```python
from build123d import *

# Parameters (mm, degrees)
SKETCH1_W           = 384
SKETCH1_H           = 140
SKETCH1_R           = 4
SKETCH1_R_2         = 3
BOSS_EXTRUDE1_DEPTH = 3
FILLET1_R           = 3


with BuildPart() as part:
    # Sketch1 → Boss-Extrude1 (new body)
    with BuildSketch(Plane(origin=(0, 0, 0), x_dir=(1, 0, 0), z_dir=(0, 1, 0))):
        Rectangle(SKETCH1_W, SKETCH1_H)
        with Locations(Location((-34, 56, 0), (0, 0, 270))):
            Circle(SKETCH1_R, mode=Mode.SUBTRACT)
        with Locations(Location((-39.2, 10, 0), (0, 0, 270))):
            Circle(SKETCH1_R, mode=Mode.SUBTRACT)
        with Locations(Location((0, -56, 0), (0, 0, 270))):
            Circle(SKETCH1_R, mode=Mode.SUBTRACT)
        with Locations(Location((39.2, 10, 0), (0, 0, 90))):
            Circle(SKETCH1_R, mode=Mode.SUBTRACT)
        with Locations(Location((34, 56, 0), (0, 0, 90))):
            Circle(SKETCH1_R, mode=Mode.SUBTRACT)
        with Locations(Location((-178, -56, 0), (0, 0, 270))):
            Circle(SKETCH1_R_2, mode=Mode.SUBTRACT)
        with Locations(Location((178, -56, 0), (0, 0, 90))):
            Circle(SKETCH1_R_2, mode=Mode.SUBTRACT)
        with Locations(Location((-178, 56, 0), (0, 0, 90))):
            Circle(SKETCH1_R_2, mode=Mode.SUBTRACT)
        with Locations(Location((178, 56, 0), (0, 0, 270))):
            Circle(SKETCH1_R_2, mode=Mode.SUBTRACT)
        with Locations(Location((-178, 18.666666667, 0), (0, 0, 270))):
            Circle(SKETCH1_R_2, mode=Mode.SUBTRACT)
        with Locations(Location((-178, -18.666666667, 0), (0, 0, 90))):
            Circle(SKETCH1_R_2, mode=Mode.SUBTRACT)
        with Locations(Location((178, 18.666666667, 0), (0, 0, 90))):
            Circle(SKETCH1_R_2, mode=Mode.SUBTRACT)
        with Locations(Location((178, -18.666666667, 0), (0, 0, 270))):
            Circle(SKETCH1_R_2, mode=Mode.SUBTRACT)
        with BuildLine():
            Line((-28.508169209, 15.556618484), (-26.070198724, 37.123280462))
            ThreePointArc((-26.070198724, 37.123280462), (-22.795588541, 43.457640532), (-16.133486944, 46))
            Line((-16.133486944, 46), (16.133486944, 46))
            ThreePointArc((16.133486944, 46), (22.795588541, 43.457640532), (26.070198724, 37.123280462))
            Line((26.070198724, 37.123280462), (28.508169209, 15.556618484))
            ThreePointArc((28.508169209, 15.556618484), (28.348223714, 12.33218572), (27.169289942, 9.326746589))
            Line((27.169289942, 9.326746589), (8.597832514, -21.941523571))
            ThreePointArc((8.597832514, -21.941523571), (0, -26.834932138), (-8.597832514, -21.941523571))
            Line((-8.597832514, -21.941523571), (-27.169289942, 9.326746589))
            ThreePointArc((-27.169289942, 9.326746589), (-28.348223714, 12.33218572), (-28.508169209, 15.556618484))
        make_face(mode=Mode.SUBTRACT)
    extrude(amount=BOSS_EXTRUDE1_DEPTH)

    # Fillet1
    fillet1_edges = [part.edges().sort_by_distance(p)[0] for p in [
        (192, 1.5, 70),
        (-192, 1.5, 70),
        (-192, 1.5, -70),
        (192, 1.5, -70),
    ]]
    fillet(fillet1_edges, radius=FILLET1_R)


solid = part.part
```
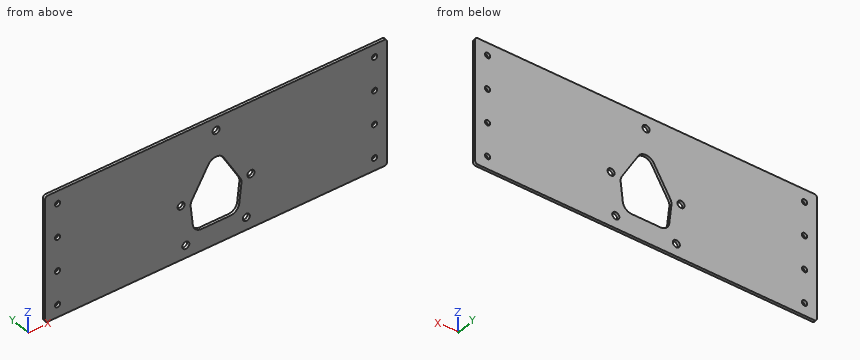
Can you work these out from the model? Positions are in its coordinate system, mm. Coordinates: 2 decimals unless noted, no trailing zeros. Write each loop counter-clockwise with the first axis right and the second up, starting at its lowest first coordinate (ties: lowest second). Pieces come first, ordered by that corner, then holes. Notation, with made-up numbers: M 76.25,18.25 L 93.25,18.25 A37 ccw 93.25,56.25 Z; hole C 74,74 d9. An arc over 180 degrees is marked long. Write item = value, one per line. Start each with the question number.
Q1. If I drill on L1, parallel to Z at x = 0.5, y = 0.3; L2, parallel to Z at x = 178, y = 1.8; L3, parallel to X at y = 1.95, z = -56, over which ranges is the centre line in solid material (lowest first)? Write a range as [from, to].
Q2. I'm going to push a flat-ended pin straight in: pin 1 (6.5 mm diameter, centred on x = -39.2, z = -10, fed in from -Y). Where does the tip first touch, or does it pass through?
Q3. If we section it at C-C, the plane z = 9: Write out the boundary of the cut face in (x, y), then the cut area to 3 significant figures.
Q4. If we section it at A-A, the plane x = 0: Write out the boundary of the cut face in (y, z), then the cut area to 3 significant figures.
Q5. If we section it at B-B, the plane y = 0.6: State how many separate pieces and enclosed holes the cut face has, then the cut area to 3 significant figures.
Check sheet entries:
q1.L1 = [-70, -46], [26.82, 52.03], [59.97, 70]
q1.L2 = [-70, -59], [-53, -21.67], [-15.67, 15.67], [21.67, 53], [59, 70]
q1.L3 = [-192, -181], [-175, -38], [-30, 30], [38, 175], [181, 192]
q2.pin_1 = through
q3.outline = M -192,0 L -16.28,0 L -16.28,3 L -192,3 Z; M 16.28,0 L 192,0 L 192,3 L 16.28,3 Z
q3.area = 1,050 mm²
q4.outline = M 0,-70 L 3,-70 L 3,-46 L 0,-46 Z; M 0,26.83 L 3,26.83 L 3,52 L 0,52 Z; M 0,60 L 3,60 L 3,70 L 0,70 Z
q4.area = 177 mm²
q5.separate_pieces = 1
q5.enclosed_holes = 14
q5.area = 50,100 mm²
